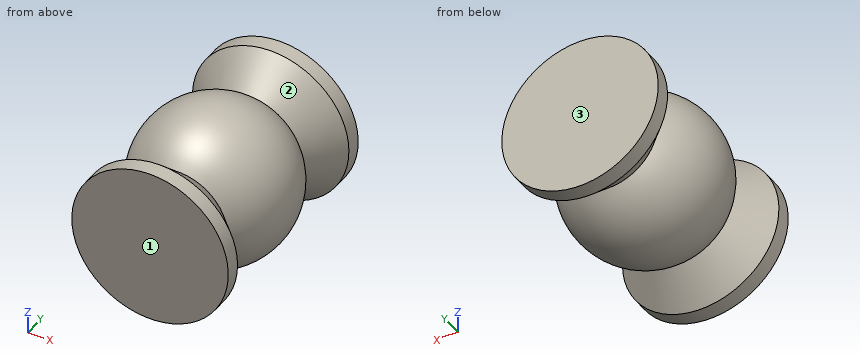
from build123d import *

# Parameters (mm, degrees)
SKETCH_1_R      = 25
EXTRUDE_1_DEPTH = 5


with BuildPart() as part:
    # 草图1 → 凸台-拉伸1 (new body)
    with BuildSketch(Plane(origin=(0, 0, 0), x_dir=(1, 0, 0), z_dir=(0, 1, 0))):
        with Locations(Location((0, 0, 0), (0, 0, 270))):
            Circle(SKETCH_1_R)
    extrude_1 = extrude(amount=-EXTRUDE_1_DEPTH)

    # 草图9 → 旋转20 (revolve)
    with BuildSketch(Plane.XY):
        with BuildLine():
            Line((15.572827559, -15.442724069), (25, -5))
            Line((25, -5), (0, -5))
            Line((0, -5), (0, -65))
            Line((0, -65), (25, -65))
            Line((25, -65), (15.572827559, -54.557275931))
            ThreePointArc((15.572827559, -54.557275931), (25, -35), (15.572827559, -15.442724069))
        make_face()
    revolve(axis=Axis((0, 51.125830707, 0), (0, -1, 0)))

    # 镜向1: 凸台-拉伸1 across plane
    add(extrude_1.mirror(Plane.ZX.offset(-35)))


solid = part.part
CAD build for the part. Positions are in the model's coordinates, mm. Face numbers are marked on the shaded views. Round coordinates to 2 decimals unless told otherwise and drop trailing zeros. Write each loop counter-clockwise with the first axis right and the second up, starting at its lowest first coordinate (ties: lowest second). Pieces come first, ordered by that corner, then holes. Notation, with made-up numbers: M 53.25,-4.5 L 60.25,-4.5 A36 cw 60.25,34.5 Z; hole C -21,73.25 d11. An arc over 180 degrees is marked long. Put each result on its own line as item: value. Start each with the question number.
1) Saw through at B-B, the plane x = 0. Write the cut outline in (y, z).
2) Saw through at A-A, the plane z = 0. Write the cut outline in (x, y), and give its area (3 significant figures).
3) Saw through at C-C, the plane z = -20. Count the separate pieces of the cut face and the enclosed holes in it, and give its area (3 significant figures).
4) Pin check, flat tips, straight feed: pin 1 Ø12 at (y, z) = (-34.5, 6.5) entering from +X; pin 2 Ø2 at (y, z) = (-24, 19) entering from -X; pin 3 Ø3 at (x, y) = (-14.5, -14.5) entering from -Z. Stop position of each tip, or through.
5) Drill centre lines: probe 1 along Y at (x, z) = (9.5, -15); probe 2 along Y at (x, z) = (-2, 17); probe 3 along Z at (x, y) = (9, -59.5). Where is each one in solid material? Low to high. Write a range as [from, to].
6) Pull direction Y, two halves, no side cores. Call the marked faces 1, 2 and 3: pulls with the +Y half, pulls with the -Y half, needs draft (parallel to the pull), parting line crosses it, or undercut.
Resolved:
1. outline: M -70,-25 L -65,-25 L -54.56,-15.57 A25 ccw -15.44,-15.57 L -5,-25 L 0,-25 L 0,25 L -5,25 L -15.44,15.57 A25 ccw -54.56,15.57 L -65,25 L -70,25 Z
2. outline: M -25,-70 L 25,-70 L 25,-65 L 15.57,-54.56 A25 ccw 15.57,-15.44 L 25,-5 L 25,0 L -25,0 L -25,-5 L -15.57,-15.44 A25 ccw -15.57,-54.56 L -25,-65 Z
2. area: 3,080 mm²
3. separate pieces: 3
3. enclosed holes: 0
3. area: 1,220 mm²
4. pin 1: x = 24.99
4. pin 2: x = -13.63
4. pin 3: z = -11.03
5. probe 1: [-70, -56.97], [-52.6, -17.4], [-13.03, 0]
5. probe 2: [-70, -56.27], [-53.22, -16.78], [-13.73, 0]
5. probe 3: [-17.9, 17.9]
6. face 1: pulls with the -Y half
6. face 2: undercut
6. face 3: pulls with the +Y half
